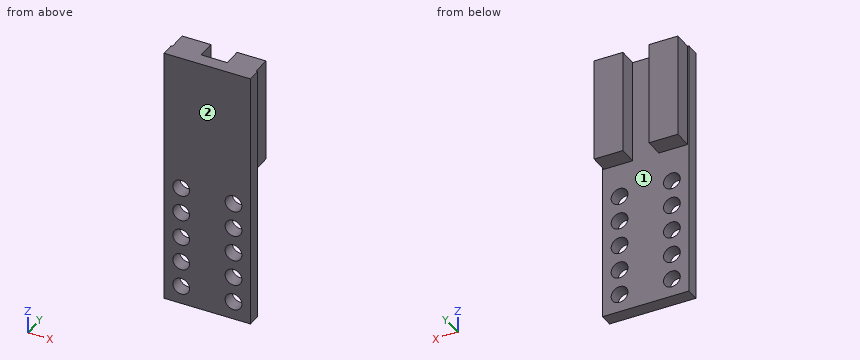
```python
from build123d import *

# Parameters (mm, degrees)
SKETCH1_W           = 16.5
SKETCH1_H           = 50
BOSS_EXTRUDE1_DEPTH = 2.5
SKETCH2_W           = 5.5
SKETCH2_H           = 20.032642475
BOSS_EXTRUDE2_DEPTH = 3.5
SKETCH4_R           = 1.6
CUT_EXTRUDE1_DEPTH  = 3.5
LPATTERN1_COUNT     = 5
LPATTERN1_PITCH     = 5


with BuildPart() as part:
    # Sketch1 → Boss-Extrude1 (new body)
    with BuildSketch(Plane(origin=(0, 0, 0), x_dir=(1, 0, 0), z_dir=(0, 1, 0))):
        Rectangle(SKETCH1_W, SKETCH1_H)
    extrude(amount=-BOSS_EXTRUDE1_DEPTH)

    # Sketch2 → Boss-Extrude2 (add)
    with BuildSketch(Plane(origin=(0, 0, 0), x_dir=(1, 0, 0), z_dir=(0, 1, 0))):
        with Locations((-5.25, -14.983678763)):
            Rectangle(SKETCH2_W, SKETCH2_H)
        with Locations((5.25, -14.983678763)):
            Rectangle(SKETCH2_W, SKETCH2_H)
    extrude(amount=BOSS_EXTRUDE2_DEPTH)

    # Sketch4 → Cut-Extrude1 (cut, through all)
    with BuildSketch(Plane(origin=(0, 0, 0), x_dir=(1, 0, 0), z_dir=(0, 1, 0))):
        with Locations((-5, 21.5)):
            Circle(SKETCH4_R)
        with Locations((5, 21.5)):
            Circle(SKETCH4_R)
    cut_extrude1 = extrude(amount=-CUT_EXTRUDE1_DEPTH, mode=Mode.SUBTRACT)

    # LPattern1: Cut-Extrude1 ×5
    with Locations(*[(0, 0, i * LPATTERN1_PITCH) for i in range(1, LPATTERN1_COUNT)]):
        add(cut_extrude1, mode=Mode.SUBTRACT)


solid = part.part
```
Source: CAD feature listing. Evaluate the final solid. Frame: model axes, mm. Face numbers are marked on the shaded views. Round coordinates to 2 decimals unless told otherwise and drop trailing zeros. Loops run counter-clockwise (first coordinate to the right, second up) from the corner with the lowest first, then second, coordinate; pieces in that order, holes last. Notation, with made-up numbers: M -12.5,57 L 46.5,57 A29 cw 46.5,93 Z; hole C -35,-1 d1. An arc over 180 degrees is marked long. Put each result on its own line as item: value.
(1) Section D-D, the plane x = 4.5. Return loops of the section in (y, z).
Solutions:
outline: M -2.5,-25 L 0,-25 L 0,-23.02 L -2.5,-23.02 Z; M -2.5,-19.98 L 0,-19.98 L 0,-18.02 L -2.5,-18.02 Z; M -2.5,-14.98 L 0,-14.98 L 0,-13.02 L -2.5,-13.02 Z; M -2.5,-9.98 L 0,-9.98 L 0,-8.02 L -2.5,-8.02 Z; M -2.5,-4.98 L 0,-4.98 L 0,-3.02 L -2.5,-3.02 Z; M -2.5,0.02 L 0,0.02 L 0,4.97 L 3.5,4.97 L 3.5,25 L -2.5,25 Z
(2) First-contact query: pin 1 (1.8 mm diameter, centred on y = 1.5, z = 18, fed in from -X); pin 2 (2 mm diameter, centred on x = -2.5, z = -9.5, fed in from +Y); pin 3 (1.8 mm diameter, centred on x = 6, y = 1.5, fed in from -Z). Flat tips, straight axial feed; report the tip coordinate or a pass-through.
Solutions:
pin 1: x = -8
pin 2: y = 0
pin 3: z = 4.97
(3) Section C-C, the plane z = -21.5. Return loops of the section in (x, y), and give its area (4 significant figures).
Solutions:
outline: M -8.25,-2.5 L -6.6,-2.5 L -6.6,0 L -8.25,0 Z; M -3.4,-2.5 L 3.4,-2.5 L 3.4,0 L -3.4,0 Z; M 6.6,-2.5 L 8.25,-2.5 L 8.25,0 L 6.6,0 Z
area: 25.25 mm²
(4) Section B-B, the plane y = 0.6. Return loops of the section in (x, z), and give its area (3 significant figures).
Solutions:
outline: M -8,4.97 L -2.5,4.97 L -2.5,25 L -8,25 Z; M 2.5,4.97 L 8,4.97 L 8,25 L 2.5,25 Z
area: 220 mm²
(5) Section A-A, the plane x = -5. Return loops of the section in (y, z), and give its area (3 significant figures).
Solutions:
outline: M -2.5,-25 L 0,-25 L 0,-23.1 L -2.5,-23.1 Z; M -2.5,-19.9 L 0,-19.9 L 0,-18.1 L -2.5,-18.1 Z; M -2.5,-14.9 L 0,-14.9 L 0,-13.1 L -2.5,-13.1 Z; M -2.5,-9.9 L 0,-9.9 L 0,-8.1 L -2.5,-8.1 Z; M -2.5,-4.9 L 0,-4.9 L 0,-3.1 L -2.5,-3.1 Z; M -2.5,0.1 L 0,0.1 L 0,4.97 L 3.5,4.97 L 3.5,25 L -2.5,25 Z
area: 155 mm²
(6) Ray query, line 1 (X direction, y = -0.65, z = -21.5); line 2 (Z direction, x = -5, y = -1.95); line 3 (X direction, y = 0.25, z = 13.5). Return the intervals inside material, ascending. Write a range as [from, to].
Solutions:
line 1: [-8.25, -6.6], [-3.4, 3.4], [6.6, 8.25]
line 2: [-25, -23.1], [-19.9, -18.1], [-14.9, -13.1], [-9.9, -8.1], [-4.9, -3.1], [0.1, 25]
line 3: [-8, -2.5], [2.5, 8]
(7) Pull-direction query (X, two-part tool) for the marked faces 1 and 2; classes: released by +X, released by -X, zero draft, split by the parting line, or undercut.
Solutions:
face 1: undercut
face 2: zero draft
